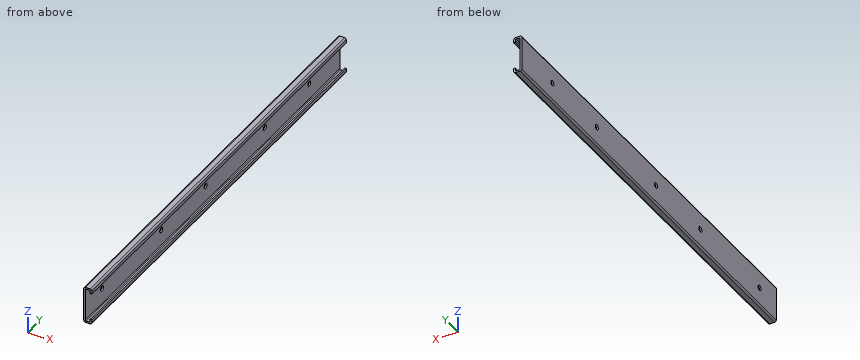
from build123d import *

# Parameters (mm, degrees)
F1_DEPTH = 550
F2_R     = 3.2
F3_DEPTH = 2


with BuildPart() as f1:
    # F0 (on Front) → F1 (new body)
    with BuildSketch(Plane.XZ):
        with BuildLine():
            ThreePointArc((0, 2), (0.585786, 0.585786), (2, 0))
            Line((2, 0), (8, 0))
            ThreePointArc((8, 0), (9.414214, 0.585786), (10, 2))
            Line((10, 2), (10, 6))
            Line((10, 6), (8, 6))
            Line((8, 6), (8, 3))
            ThreePointArc((8, 3), (7.707107, 2.292893), (7, 2))
            Line((7, 2), (3, 2))
            ThreePointArc((3, 2), (2.292893, 2.292893), (2, 3))
            Line((2, 3), (2, 42.2))
            ThreePointArc((2, 42.2), (2.292893, 42.907107), (3, 43.2))
            Line((3, 43.2), (7, 43.2))
            ThreePointArc((7, 43.2), (7.707107, 42.907107), (8, 42.2))
            Line((8, 42.2), (8, 39.2))
            Line((8, 39.2), (10, 39.2))
            Line((10, 39.2), (10, 43.2))
            ThreePointArc((10, 43.2), (9.414214, 44.614214), (8, 45.2))
            Line((8, 45.2), (2, 45.2))
            ThreePointArc((2, 45.2), (0.585786, 44.614214), (0, 43.2))
            Line((0, 43.2), (0, 2))
        make_face()
    extrude(amount=-F1_DEPTH)

    # F2 (on face) → F3 (cut)
    with BuildSketch(Plane(origin=(0, 0, 0), x_dir=(0, -1, 0), z_dir=(-1, 0, 0))):
        with Locations((-36, 22.6)):
            Circle(F2_R)
        with Locations((-164, 22.6)):
            Circle(F2_R)
        with Locations((-260, 22.6)):
            Circle(F2_R)
        with Locations((-388, 22.6)):
            Circle(F2_R)
        with Locations((-484, 22.6)):
            Circle(F2_R)
    extrude(amount=-F3_DEPTH, mode=Mode.SUBTRACT)


solid = f1.part
The listing builds one solid part. Answer for the finished solid, in the listing's coordinates (mm). Give positions to 0.01 mm unless a question says otherwise; leave off trailing zeros. Write each loop counter-clockwise with the first axis right and the second up, starting at its lowest first coordinate (ties: lowest second). Pieces come first, ordered by that corner, then holes.
1) Section A-A (y = 183.5) is taken. Write down the section's boundary in (x, z).
2) Section B-B (z = 33) is taken. Write down the section's boundary in (x, y).
3) Given P1, Ø1.5, axis at y = 195.5, z = 5, coming from the -X side; P2, Ø4, axis at y = 260, z = 22.6, coming from the -X side; P3, Ø3, axis at y = 245, z = 9, coming from the +X side; P4, Ø1, axis at x = 9, y = 342, coming from the +Z side, each flat-ended and moving along its own axis, determine where each tip first touches the part or whether it passes through.
4) Find the intervals of material crossed by L1, parallel to Z at x = 5, y = 91.5; L2, parallel to X at y = 32.5, z = 42; L3, parallel to X at y = 233.5, z = 30, in increasing order.
Response:
1. outline: (0, 2) arc R2 ccw to (2, 0) - (8, 0) arc R2 ccw to (10, 2) - (10, 6) - (8, 6) - (8, 3) arc R1 cw to (7, 2) - (3, 2) arc R1 cw to (2, 3) - (2, 42.2) arc R1 cw to (3, 43.2) - (7, 43.2) arc R1 cw to (8, 42.2) - (8, 39.2) - (10, 39.2) - (10, 43.2) arc R2 ccw to (8, 45.2) - (2, 45.2) arc R2 ccw to (0, 43.2) - close
2. outline: (0, 0) - (2, 0) - (2, 550) - (0, 550) - close
3. P1: stops at x = 0
3. P2: passes through
3. P3: stops at x = 2
3. P4: stops at z = 45.14
4. L1: z = 0 to 2, 43.2 to 45.2
4. L2: x = 0 to 2, 8 to 10
4. L3: x = 0 to 2
